Verification items for the finished model (mm, model axes). A direction names the side the tool comes from. Give positions to 0.01 mm unless a question says otherwise; leave off trailing zeros. Write each loop counter-clockwise with the first axis right and the second up, starting at its lowest first coordinate (ties: lowest second). Pieces come first, ordered by that corner, then holes. Notation, with made-up numbers: (20.25, 79) -> (66.25, 79) arc R27 ccw to (66.25, 116) -> close; hole circle Ø9 at (-18.5, 20). An arc over 180 degrees is marked (long way). Use CSV: the item, a comma, the result in double quotes. Start each with the question number.
```python
from build123d import *

# Parameters (mm, degrees)
SKETCH1_R           = 6
BOSS_EXTRUDE1_DEPTH = 2
SKETCH2_R           = 2.7
BOSS_EXTRUDE2_DEPTH = 10
CUT_EXTRUDE1_DEPTH  = 8


with BuildPart() as part:
    # Sketch1 → Boss-Extrude1 (new body)
    with BuildSketch(Plane(origin=(0, 0, 0), x_dir=(1, 0, 0), z_dir=(0, 1, 0))):
        Circle(SKETCH1_R)
    extrude(amount=BOSS_EXTRUDE1_DEPTH)

    # Sketch2 → Boss-Extrude2 (add)
    with BuildSketch(Plane(origin=(0, 2, 0), x_dir=(1, 0, 0), z_dir=(0, 1, 0))):
        Circle(SKETCH2_R)
    extrude(amount=BOSS_EXTRUDE2_DEPTH)

    # Sketch3 → Cut-Extrude1 (cut)
    with BuildSketch(Plane(origin=(0, 12, 0), x_dir=(1, 0, 0), z_dir=(0, 1, 0))):
        with BuildLine():
            Line((-1.965, 1.851695169), (1.965, 1.851695169))
            ThreePointArc((1.965, 1.851695169), (0, 2.7), (-1.965, 1.851695169))
        make_face()
        with BuildLine():
            Line((-1.965, -1.851695169), (1.965, -1.851695169))
            ThreePointArc((1.965, -1.851695169), (0, -2.7), (-1.965, -1.851695169))
        make_face()
    extrude(amount=-CUT_EXTRUDE1_DEPTH, mode=Mode.SUBTRACT)


solid = part.part
```
(1) Thickness scan on line 1 (Z direction, x = 0, y = 11); line 2 (Y direction, x = 4.5, z = -2.5); line 3 (X direction, y = 6.75, z = -1.25). Record the ranges inside material, lowest first. Write a range as from..to.
(2) Section check D-D on x = 2.25. Record the cut outline in (y, z), then the cut area to 3 significant figures.
(3) Set-up check for faces 1 (the face through (0, 8, 1.852)), 2 (the face through (0, 0, 0)), 3 (the face through (-2.7, 5.8, -0.1)), 4 (the face through (0, 4, -2.2)): record each of +Z, -Z, +X, -X, +Y, -Y from which the full face is reachable in a straight line by a thin tool's end or side.
(4) Go/stop test with flat-tipped pins: pin 1 (3 mm diameter, centred on x = -3.5, y = 1.5, fed in from -Z); pin 2 (5 mm diameter, centred on x = 3.5, z = 2.5, fed in from -Y); pin 3 (3 mm diameter, centred on x = 0.5, y = 9, fed in from -Z); pin 4 (1.5 mm diameter, centred on x = 1, y = 3, fed in from -Z). Record where each tip stops, or that it passes through.
(5) Section check C-C on y = 3. Record the cut outline in (x, z), then the cut area to 3 significant figures.
(6) Section check B-B on z = 0. Record the cut outline in (x, y), then the cut area to 3 significant figures.
(7) Section check A-A on x = 0. Record the cut outline in (y, z), then the cut area to 3 significant figures.
Data:
1,line 1,"z = -1.85..1.85"
1,line 2,"y = 0..2"
1,line 3,"x = -2.39..2.39"
2,outline,"(0, -5.56) -> (2, -5.56) -> (2, -1.49) -> (12, -1.49) -> (12, 1.49) -> (2, 1.49) -> (2, 5.56) -> (0, 5.56) -> close"
2,area,"52.1 mm2"
3,face 1,"+Z, +X, -X, +Y"
3,face 2,"+Z, -Z, +X, -X, -Y"
3,face 3,"+Y"
3,face 4,"-Z, +X, -X, +Y"
4,pin 1,"stops at z = -5.66"
4,pin 2,"stops at y = 0"
4,pin 3,"stops at z = -1.85"
4,pin 4,"stops at z = -2.69"
5,outline,"circle Ø5.4 at (0, 0)"
5,area,"22.9 mm2"
6,outline,"(-6, 0) -> (6, 0) -> (6, 2) -> (2.7, 2) -> (2.7, 12) -> (-2.7, 12) -> (-2.7, 2) -> (-6, 2) -> close"
6,area,"78.0 mm2"
7,outline,"(0, -6) -> (2, -6) -> (2, -2.7) -> (4, -2.7) -> (4, -1.85) -> (12, -1.85) -> (12, 1.85) -> (4, 1.85) -> (4, 2.7) -> (2, 2.7) -> (2, 6) -> (0, 6) -> close"
7,area,"64.4 mm2"
